The listing builds one solid part. Answer for the finished solid, in the listing's coordinates (mm). A direction names the side the tool comes from. Coordinates: 2 decimals unless noted, no trailing zeros. Order: outer loops, then holes, each group sorted by start corner. A loop starts at its lowest first (then second) coordinate and runs counter-clockwise, first axis right, second up. Notation, with made-up numbers: M -25,-18.5 L 13,-18.5 A31 ccw 13,10.5 Z; hole C 77.5,70.25 d9. An arc over 180 degrees is marked long. One line per item, written item: value. Start each with the question number.
Q1. Straight lines are drawn through the part: line 1 along Y through (x, z) = (0.75, -2.5); line 2 along Z through (x, y) = (-1, 15.25); line 3 along X through (y, z) = (5, -3). For each, find the intervals that lie inside material, in ascending order. Write a range as [from, to].
Q2. The part is cut by section B-B on z = 0.5. Give the vertices of the cut face in (x, y).
Q3. The part is cut by section C-C on x = 1. Give the vertices of the cut face in (y, z).
Q4. For faces 1 (the cylindrical face through (0.563, 19.577, 1.787)), 2 (the flat face through (3.13, 6.9, 0.16)), determine the directions among +Z, -Z, +X, -X, +Y, -Y from which every point of the face is accessible in a straight line to the end or side of a thin tool.
Q5. The part is cut by section D-D on y = 22.25. Give the vertices of the cut face in (x, z), then the cut area to 3 significant figures.
Q6. The part is cut by section A-A on y = 12.25. Give the vertices of the cut face in (x, z).
```python
from build123d import *

# Parameters (mm, degrees)
BOSS_EXTRUDE1_DEPTH = 25
SKETCH2_OUTSIDE_W   = 13.782
SKETCH2_OUTSIDE_H   = 14.596
SKETCH2_OUTSIDE_R   = 1.873084861
CUT_EXTRUDE1_DEPTH  = 11


with BuildPart() as part:
    # Sketch1 → Boss-Extrude1 (new body)
    with BuildSketch(Plane(origin=(0, 0, 0), x_dir=(1, 0, 0), z_dir=(0, 1, 0))):
        Polygon((3.210447175, 1.67252173), (0.156777281, 3.616589676), (-3.053669894, 1.944067946), (-3.210447175, -1.67252173), (-0.156777281, -3.616589676), (3.053669894, -1.944067946), align=None)
    extrude(amount=BOSS_EXTRUDE1_DEPTH)

    # Sketch2 outside → Cut-Extrude1 (cut)
    with BuildSketch(Plane(origin=(0, 25, 0), x_dir=(1, 0, 0), z_dir=(0, 1, 0))):
        Rectangle(SKETCH2_OUTSIDE_W, SKETCH2_OUTSIDE_H)
        with Locations(Location((0, 0, 0), (0, 0, 270))):
            Circle(SKETCH2_OUTSIDE_R, mode=Mode.SUBTRACT)
    extrude(amount=-CUT_EXTRUDE1_DEPTH, mode=Mode.SUBTRACT)


solid = part.part
```
Output:
1. line 1: y = [0, 14]
1. line 2: z = [-1.58, 1.58]
1. line 3: x = [-1.03, 1.13]
2. outline: M -3.16,0 L 3.12,0 L 3.12,14 L 1.81,14 L 1.81,25 L -1.81,25 L -1.81,14 L -3.16,14 Z
3. outline: M 0,-3.08 L 14,-3.08 L 14,-1.58 L 25,-1.58 L 25,1.58 L 14,1.58 L 14,3.01 L 0,3.01 Z
4. face 1: +Y
4. face 2: +Z, +X, +Y, -Y
5. outline: C 0,0 d3.75
5. area: 11.0 mm^2
6. outline: M -3.21,1.67 L -3.05,-1.94 L 0.16,-3.62 L 3.21,-1.67 L 3.05,1.94 L -0.16,3.62 Z
